Here's how the part is built. I have some questions about the finished solid (model axes, mm). Face numbers are marked on the shaded views. A direction names the side the tool comes from. Coordinates: 2 decimals unless noted, no trailing zeros. Loops run counter-clockwise (first coordinate to the right, second up) from the corner with the lowest first, then second, coordinate; pieces in that order, holes last. Notation, with made-up numbers: M 9,84.5 L 26,84.5 A24 ccw 26,103.5 Z; hole C 8,-27.5 d9. An arc over 180 degrees is marked long. Use CSV: the item, a comma, the result in double quotes. Start each with the question number.
Q1. For pin 1 Ø1.2 at (x, y) = (-0.5, 0.5) entering from +Z; pin 2 Ø1 at (x, y) = (-1, -1) entering from -Z, each with a flat end and sliding along its axis, tell me the tip position at first contact or that it passes through.
Q2. If we section it at C-C (y = -0.5): Please give me the cut outline in (x, z), and give its area (3 significant figures).
Q3. If we mould it in two halves opening along X, with no side actions, what happens to the marked faces 4, 5 and 6? For each: +X half, -X half, draft (parallel to the pull), parting line (faces both ways), or undercut.
Q4. If we section it at B-B (x = 0): Please give me the cut outline in (y, z).
Q5. Please list where these lines run through material, in increasing order: probe 1 along Z at (x, y) = (0, -0.35); probe 2 along Y at (x, z) = (-0.8, 16.5); probe 3 along Y at (x, z) = (-2.6, 12.5). Write a range as [from, to].
Q6. Which directions (+Z, -Z, +X, -X, +Y, -Y) give clear straight access to the entire face, cutting with the end or side of a thin tool? Please do the marked faces 1, 2 and 3.
Q7. If we section it at A-A (z = 5): Please give me the cut outline in (x, y), and give its area (3 significant figures).
Q8. If we section it at D-D (z = 1.75): Please give me the cut outline in (x, y).
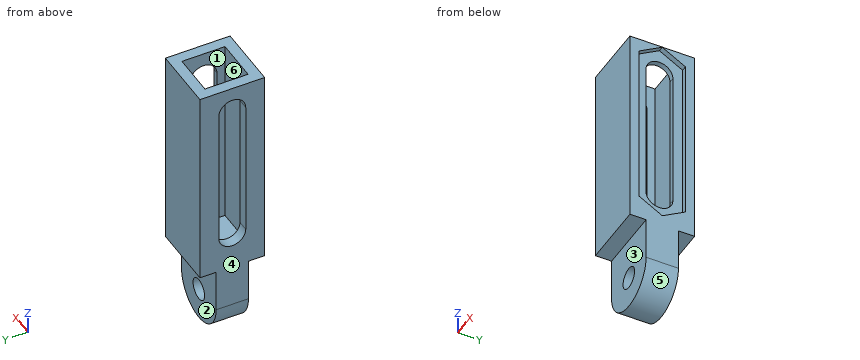
from build123d import *

# Parameters (mm, degrees)
SKETCH_1_W           = 6
SKETCH_1_H           = 6
SKETCH_1_W_2         = 4
SKETCH_1_H_2         = 4
EXTRUDE_1_DEPTH      = 18
SKETCH_2_W           = 6
SKETCH_2_H           = 6
EXTRUDE_2_DEPTH      = 1
SKETCH_3_R           = 1
EXTRUDE_3_DEPTH      = 1.5
EXTRUDE_3_DEPTH_BACK = 1.5
CUT_EXTRUDE_1_DEPTH  = 6
CUT_EXTRUDE_2_DEPTH  = 0.5


with BuildPart() as part:
    # 스케치1 → 보스-돌출1 (new body)
    with BuildSketch(Plane.XY):
        Rectangle(SKETCH_1_W, SKETCH_1_H)
        Rectangle(SKETCH_1_W_2, SKETCH_1_H_2, mode=Mode.SUBTRACT)
    extrude(amount=EXTRUDE_1_DEPTH)

    # 스케치2 → 보스-돌출2 (add)
    with BuildSketch(Plane(origin=(0, 0, 0), x_dir=(-1, 0, 0), z_dir=(0, 0, -1))):
        Rectangle(SKETCH_2_W, SKETCH_2_H)
    extrude(amount=EXTRUDE_2_DEPTH)

    # 스케치3 → 보스-돌출3 (add, two sides)
    with BuildSketch(Plane(origin=(0, 0, 0), x_dir=(1, 0, 0), z_dir=(0, 1, 0))) as extrude_3_sk:
        with BuildLine():
            Line((3, 5), (3, 1))
            Line((3, 1), (-3, 1))
            Line((-3, 1), (-3, 5))
            ThreePointArc((-3, 5), (0, 8), (3, 5))
        make_face()
        with Locations((0, 5)):
            Circle(SKETCH_3_R, mode=Mode.SUBTRACT)
    extrude(amount=EXTRUDE_3_DEPTH)
    extrude(extrude_3_sk.sketch, amount=-EXTRUDE_3_DEPTH_BACK)

    # 스케치4 → 컷-돌출1 (cut)
    with BuildSketch(Plane.ZY.offset(3)):
        with BuildLine():
            Line((15.5, 1.25), (2.5, 1.25))
            ThreePointArc((2.5, 1.25), (1.25, 0), (2.5, -1.25))
            Line((2.5, -1.25), (15.5, -1.25))
            ThreePointArc((15.5, -1.25), (16.75, 0), (15.5, 1.25))
        make_face()
    extrude(amount=-CUT_EXTRUDE_1_DEPTH, mode=Mode.SUBTRACT)

    # 스케치5 → 컷-돌출2 (cut)
    with BuildSketch(Plane(origin=(3, 0, 0), x_dir=(0, 0, -1), z_dir=(1, 0, 0))):
        Polygon((-9, 2.15), (-16.741303079, 2.15), (-17.982606158, 0), (-16.741303079, -2.15), (-9, -2.15), (-1.258696921, -2.15), (-0.017393842, 0), (-1.258696921, 2.15), align=None)
    extrude(amount=-CUT_EXTRUDE_2_DEPTH, mode=Mode.SUBTRACT)


solid = part.part
Results below:
1,pin 1,"z = 0"
1,pin 2,"z = -7.96"
2,outline,"M -3,-5 A3 ccw 3,-5 L 3,0.31 L 2.5,0.31 L 2.5,1.35 L 2,1.35 L 2,0 L -2,0 L -2,1.35 L -3,1.35 Z; M -3,16.65 L -2,16.65 L -2,18 L -3,18 Z; M 2,16.65 L 2.5,16.65 L 2.5,17.69 L 3,17.69 L 3,18 L 2,18 Z; hole C 0,-5 d2"
2,area,"45.4 mm^2"
3,face 4,"-X half"
3,face 5,"parting line"
3,face 6,"undercut"
4,outline,"M -3,-1 L -1.5,-1 L -1.5,-4 L 1.5,-4 L 1.5,-1 L 3,-1 L 3,18 L 2,18 L 2,0 L -2,0 L -2,18 L -3,18 Z; M -1.5,-8 L 1.5,-8 L 1.5,-6 L -1.5,-6 Z"
5,probe 1,"[-8, -6], [-4, 0]"
5,probe 2,"[-3, -2], [2, 3]"
5,probe 3,"[-3, -1.25], [1.25, 3]"
6,face 1,"+Z"
6,face 2,"-Z, +X, -X, +Y"
6,face 3,"-Z, +X, -X, -Y"
7,outline,"M -3,-3 L 3,-3 L 3,-2.15 L 2.5,-2.15 L 2.5,-1.25 L 2,-1.25 L 2,-2 L -2,-2 L -2,-1.25 L -3,-1.25 Z; M -3,1.25 L -2,1.25 L -2,2 L 2,2 L 2,1.25 L 2.5,1.25 L 2.5,2.15 L 3,2.15 L 3,3 L -3,3 Z"
7,area,"14.1 mm^2"
8,outline,"M -3,-3 L 3,-3 L 3,-2.15 L 2.5,-2.15 L 2.5,-1 L 2,-1 L 2,-2 L -2,-2 L -2,-1 L -3,-1 Z; M -3,1 L -2,1 L -2,2 L 2,2 L 2,1 L 2.5,1 L 2.5,2.15 L 3,2.15 L 3,3 L -3,3 Z"
